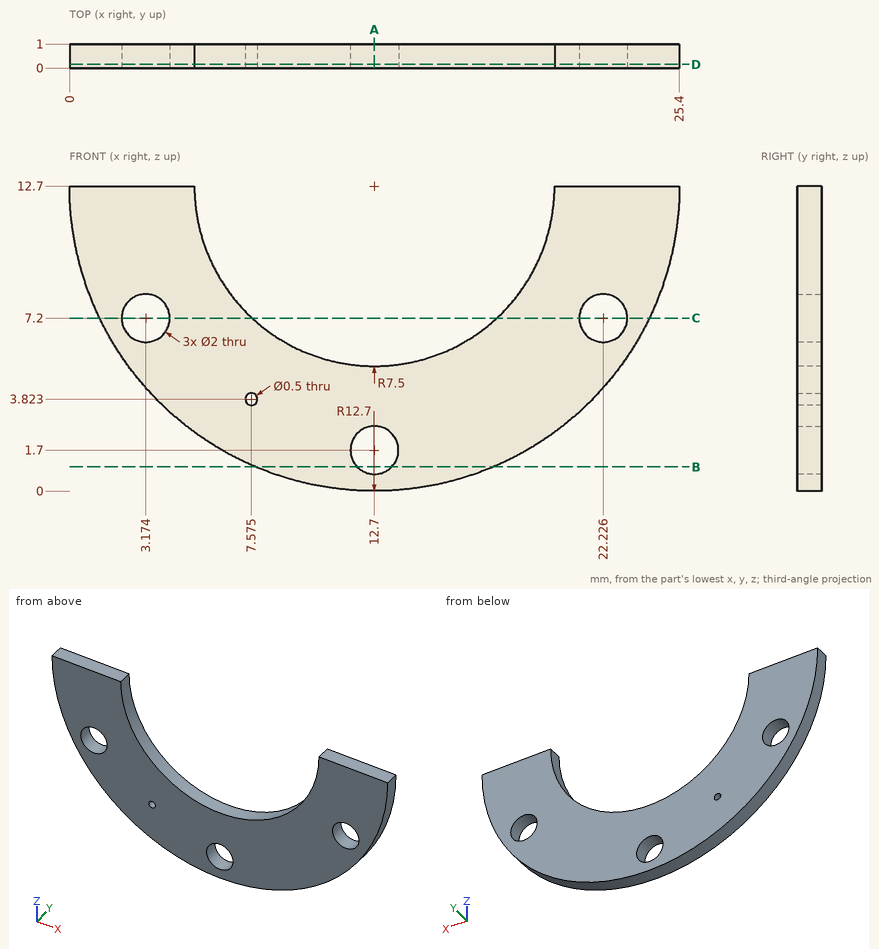
Print and shaded views of the part. All mm, measured from the part's lowest x, y and z. Round coordinates to 2 decimals unless told otherwise and drop trailing zeros. Write each loop counter-clockwise with the first axis right and the second up, starting at its lowest first coordinate (ties: lowest second). Pieces come first, ordered by that corner, then holes.
(1) Slice it at C-C, the plane z = 7.2. Write the cut outline in (x, y).
(2) Slice it at A-A, the plane x = 12.7. Write the cut outline in (y, z).
(3) Probe line 1 along Z through (x, y) = (12.7, 0.55); line 2 along X through (y, z) = (0.7, 7.2) (1 decimal); line 3 along X through (y, z) = (0.75, 6.75) (1 decimal). List the from-to ranges inside material, lowest first.
(4) Slice it at D-D, the plane y = 0.15. Count the separate pieces of the cut face and the enclosed holes in it, and give its area (3 significant figures).
(5) Slice it at B-B, the plane z = 1. Write the cut outline in (x, y).
(6) Drop a flat-ended pin along its axis: P1, Ø2.5, axis at x = 3.17, z = 7.2, coming from the +Y side. Give the stop position or say it passes through.
From the geometry:
1. outline: (1.25, 0) - (2.17, 0) - (2.17, 1) - (1.25, 1) - close; (4.17, 0) - (7.6, 0) - (7.6, 1) - (4.17, 1) - close; (17.8, 0) - (21.23, 0) - (21.23, 1) - (17.8, 1) - close; (23.23, 0) - (24.15, 0) - (24.15, 1) - (23.23, 1) - close
2. outline: (0, 0) - (1, 0) - (1, 0.7) - (0, 0.7) - close; (0, 2.7) - (1, 2.7) - (1, 5.2) - (0, 5.2) - close
3. line 1: z = 0 to 0.7, 2.7 to 5.2
3. line 2: x = 1.3 to 2.2, 4.2 to 7.6, 17.8 to 21.2, 23.2 to 24.1
3. line 3: x = 1.5 to 2.3, 4.1 to 8.1, 17.3 to 21.3, 23.1 to 23.9
4. separate pieces: 1
4. enclosed holes: 4
4. area: 155 mm2
5. outline: (7.76, 0) - (11.99, 0) - (11.99, 1) - (7.76, 1) - close; (13.41, 0) - (17.64, 0) - (17.64, 1) - (13.41, 1) - close
6. P1: stops at y = 1
